Input: part model. Units: mm. Frame: model coordinates. Face numbers are marked on the shaded views. A direction names the side the tool comes from. Round coordinates to 2 decimals unless told otherwise and drop trailing zeros. Loops run counter-clockwise (first coordinate to the right, second up) from the corner with the lowest first, then second, coordinate; pieces in that order, holes last. Notation, with made-up numbers: (5.25, 81.25) -> (15.25, 81.25) arc R26 ccw to (15.25, 100.25) -> close; hole circle Ø11 at (-22.75, -33.75). An arc over 180 degrees is marked (long way). One line per question, with ' | ' between items. Start each with the question number.
Q1. Material intervals for L1, parallel to Y at x = 0, z = 3.7; L2, parallel to Y at x = 4, z = 0.9; L3, parallel to Y at x = 2.25, z = 5.3, sorted ascending.
Q2. Access query for the marked faces 5, 6 and 7. Directions: +Z, -Z, +X, -X, +Y, -Y. A direction counts if a zero-diameter tool reaches every point of the face in a straight line with its end or side. Return the directions, or none.
Q3. Contact query for flat-ended pins moving along their axis: P1, Ø1, axis at y = 3, z = 1.5, coming from the -X side; P2, Ø1.4, axis at x = 8.5, z = 3, coming from the -Y side; P3, Ø3, axis at x = -5, z = 5.5, coming from the -Y side. Output: stop coordinate, or through.
Q4. Cut plane B-B on y = 4. Return loops of the section in (x, z), and give its area (3 significant figures).
Q5. Mould query, pull axis Y, two halves, no side actions, for the marked faces 1, 2, 3 and 4. Classes: pulls with the +Y half, pulls with the -Y half, needs draft (parallel to the pull), parting line crosses it, or undercut.
Q6. Cut plane A-A on x = 0. Return loops of the section in (y, z), and give its area (3 significant figures).
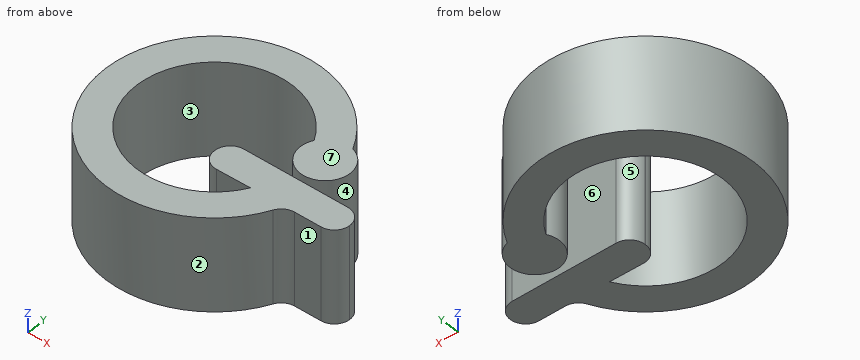
from build123d import *

# Parameters (mm, degrees)
F1_DEPTH = 6
F2_R     = 0.99999


# Not quite as in the source:
# - a fillet or chamfer is up to 0.001 mm smaller than in the source, because OpenCascade refuses the exact size


with BuildPart() as f1:
    # F0 (on Top) → F1 (new body)
    with BuildSketch(Plane.XY):
        with BuildLine():
            ThreePointArc((4.411359383, -2.3537009993), (-4.9996939131, -0.0553242752), (4.3581956764, 2.4507407954))
            ThreePointArc((4.3581956764, 2.4507407954), (6.3660027692, 0.1987741987), (6.2194307383, 3.2122704263))
            ThreePointArc((6.2194307383, 3.2122704263), (-6.9833792075, -0.482094228), (6.6018426545, -2.3271599784))
            Line((6.6018426545, -2.3271599784), (9.9892851541, -2.3271599784))
            Line((9.9892851541, -2.3271599784), (9.9892851541, -0.3271599784))
            Line((9.9892851541, -0.3271599784), (4.9892851541, -0.3271599784))
            Line((4.9892851541, -0.3271599784), (1.1988097103, -0.3271599784))
            Line((1.1988097103, -0.3271599784), (1.1988097103, -2.3926259018))
            Line((1.1988097103, -2.3926259018), (4.411359383, -2.3537009993))
        make_face()
    extrude(amount=F1_DEPTH)

    # F2 (radius 1 in the source; OpenCascade refuses exactly that, so slightly less here)
    f2_edges = [f1.edges().sort_by_distance(p)[0] for p in [
        (9.989285, -0.32716, 3),
        (1.19881, -0.32716, 3),
        (1.19881, -2.392626, 3),
        (9.989285, -2.32716, 3),
        (6.601843, -2.32716, 3),
    ]]
    fillet(f2_edges, radius=F2_R)


solid = f1.part
Results:
1) L1: -7 to -5, 5 to 7 | L2: -5.74 to -3, -2.36 to -0.33, 3 to 5.74 | L3: -6.63 to -4.47, -2.38 to -0.33, 4.47 to 6.63
2) face 5: +Z, -Z | face 6: +Z, -Z, +X | face 7: +Z, +X, -X, +Y, -Y
3) P1: x = -6.54 | P2: y = -2.33 | P3: y = -6.06
4) outline: (-5.74, 0) -> (-3, 0) -> (-3, 6) -> (-5.74, 6) -> close; (3, 0) -> (5.74, 0) -> (5.74, 6) -> (3, 6) -> close | area: 32.9 mm^2
5) face 1: pulls with the -Y half | face 2: parting line crosses it | face 3: undercut | face 4: undercut
6) outline: (-7, 0) -> (-5, 0) -> (-5, 6) -> (-7, 6) -> close; (5, 0) -> (7, 0) -> (7, 6) -> (5, 6) -> close | area: 24.0 mm^2
